```python
from build123d import *

# Parameters (mm, degrees)
SKETCH1_R           = 6
SKETCH1_R_2         = 1.1
BOSS_EXTRUDE1_DEPTH = 2.9
SKETCH2_R           = 6
CUT_EXTRUDE1_DEPTH  = 11.278132126
CUT_EXTRUDE2_DEPTH  = 2.8


with BuildPart() as part:
    # Sketch1 → Boss-Extrude1 (new, symmetric)
    with BuildSketch(Plane.XY):
        Circle(SKETCH1_R)
        Circle(SKETCH1_R_2, mode=Mode.SUBTRACT)
    extrude(amount=BOSS_EXTRUDE1_DEPTH, both=True)

    # Sketch2 → Cut-Extrude1 (cut, through all)
    with BuildSketch(Plane.XY.offset(2.9)):
        Circle(SKETCH2_R)
        with BuildLine():
            ThreePointArc((-0.904303163, 2.859411966), (-1.23929318, 3.784776039), (-2.052505646, 4.339034521))
            ThreePointArc((-2.052505646, 4.339034521), (-2.138842368, 4.297133152), (-2.224324134, 4.253514094))
            ThreePointArc((-2.224324134, 4.253514094), (-2.272407373, 3.270556831), (-1.736096974, 2.44539737))
            ThreePointArc((-1.736096974, 2.44539737), (-2.100579038, 2.140459929), (-2.412316811, 1.781776811))
            ThreePointArc((-2.412316811, 1.781776811), (-3.227244783, 2.333509881), (-4.210932449, 2.303920118))
            ThreePointArc((-4.210932449, 2.303920118), (-4.256151318, 2.219273746), (-4.29966888, 2.133740266))
            ThreePointArc((-4.29966888, 2.133740266), (-3.760801254, 1.310248516), (-2.841900466, 0.957915832))
            ThreePointArc((-2.841900466, 0.957915832), (-2.957534919, 0.496979078), (-2.998907428, 0.023563475))
            ThreePointArc((-2.998907428, 0.023563475), (-3.982498568, -0.009077739), (-4.760926181, -0.611213463))
            ThreePointArc((-4.760926181, -0.611213463), (-4.747755125, -0.706272801), (-4.732686255, -0.801049821))
            ThreePointArc((-4.732686255, -0.801049821), (-3.812696882, -1.150530198), (-2.862194572, -0.895456995))
            ThreePointArc((-2.862194572, -0.895456995), (-2.684812984, -1.336330888), (-2.440017337, -1.743650307))
            ThreePointArc((-2.440017337, -1.743650307), (-3.216573261, -2.348197971), (-3.49240793, -3.292884275))
            ThreePointArc((-3.49240793, -3.292884275), (-3.425877845, -3.362047143), (-3.357978338, -3.429866103))
            ThreePointArc((-3.357978338, -3.429866103), (-2.408271889, -3.171845481), (-1.789227635, -2.406795685))
            ThreePointArc((-1.789227635, -2.406795685), (-1.386583742, -2.659207876), (-0.949123556, -2.844848937))
            ThreePointArc((-0.949123556, -2.844848937), (-1.222026295, -3.79038639), (-0.889908552, -4.716785215))
            ThreePointArc((-0.889908552, -4.716785215), (-0.795431669, -4.733633748), (-0.700636829, -4.74859011))
            ThreePointArc((-0.700636829, -4.74859011), (-0.083968889, -3.981623598), (-0.032836554, -2.998820228))
            ThreePointArc((-0.032836554, -2.998820228), (0.44127336, -2.966357838), (0.904303163, -2.859411966))
            ThreePointArc((0.904303163, -2.859411966), (1.23929318, -3.784776039), (2.052505646, -4.339034521))
            ThreePointArc((2.052505646, -4.339034521), (2.138842368, -4.297133152), (2.224324134, -4.253514094))
            ThreePointArc((2.224324134, -4.253514094), (2.272407373, -3.270556831), (1.736096974, -2.44539737))
            ThreePointArc((1.736096974, -2.44539737), (2.100579038, -2.140459929), (2.412316811, -1.781776811))
            ThreePointArc((2.412316811, -1.781776811), (3.227244783, -2.333509881), (4.210932449, -2.303920118))
            ThreePointArc((4.210932449, -2.303920118), (4.256151318, -2.219273746), (4.29966888, -2.133740266))
            ThreePointArc((4.29966888, -2.133740266), (3.760801254, -1.310248516), (2.841900466, -0.957915832))
            ThreePointArc((2.841900466, -0.957915832), (2.957534919, -0.496979078), (2.998907428, -0.023563475))
            ThreePointArc((2.998907428, -0.023563475), (3.982498568, 0.009077739), (4.760926181, 0.611213463))
            ThreePointArc((4.760926181, 0.611213463), (4.747755125, 0.706272801), (4.732686255, 0.801049821))
            ThreePointArc((4.732686255, 0.801049821), (3.812696882, 1.150530198), (2.862194572, 0.895456995))
            ThreePointArc((2.862194572, 0.895456995), (2.684812984, 1.336330888), (2.440017337, 1.743650307))
            ThreePointArc((2.440017337, 1.743650307), (3.216573261, 2.348197971), (3.49240793, 3.292884275))
            ThreePointArc((3.49240793, 3.292884275), (3.425877845, 3.362047143), (3.357978338, 3.429866103))
            ThreePointArc((3.357978338, 3.429866103), (2.408271889, 3.171845481), (1.789227635, 2.406795685))
            ThreePointArc((1.789227635, 2.406795685), (1.386583742, 2.659207876), (0.949123556, 2.844848937))
            ThreePointArc((0.949123556, 2.844848937), (1.222026295, 3.79038639), (0.889908552, 4.716785215))
            ThreePointArc((0.889908552, 4.716785215), (0.795431669, 4.733633748), (0.700636829, 4.74859011))
            ThreePointArc((0.700636829, 4.74859011), (0.083968889, 3.981623598), (0.032836554, 2.998820228))
            ThreePointArc((0.032836554, 2.998820228), (-0.44127336, 2.966357838), (-0.904303163, 2.859411966))
        make_face(mode=Mode.SUBTRACT)
    extrude(amount=-CUT_EXTRUDE1_DEPTH, mode=Mode.SUBTRACT)

    # Sketch3 → Cut-Extrude2 (cut)
    with BuildSketch(Plane.XY.offset(2.9)):
        with BuildLine():
            ThreePointArc((0.700636829, 4.74859011), (0.083968889, 3.981623598), (0.032836554, 2.998820228))
            ThreePointArc((0.032836554, 2.998820228), (-0.44127336, 2.966357838), (-0.904303163, 2.859411966))
            ThreePointArc((-0.904303163, 2.859411966), (-1.23929318, 3.784776039), (-2.052505646, 4.339034521))
            ThreePointArc((-2.052505646, 4.339034521), (-2.138842368, 4.297133152), (-2.224324134, 4.253514094))
            ThreePointArc((-2.224324134, 4.253514094), (-2.272407373, 3.270556831), (-1.736096974, 2.44539737))
            ThreePointArc((-1.736096974, 2.44539737), (-2.100579038, 2.140459929), (-2.412316811, 1.781776811))
            ThreePointArc((-2.412316811, 1.781776811), (-3.227244783, 2.333509881), (-4.210932449, 2.303920118))
            ThreePointArc((-4.210932449, 2.303920118), (-4.256151318, 2.219273746), (-4.29966888, 2.133740266))
            ThreePointArc((-4.29966888, 2.133740266), (-3.760801254, 1.310248516), (-2.841900466, 0.957915832))
            ThreePointArc((-2.841900466, 0.957915832), (-2.957534919, 0.496979078), (-2.998907428, 0.023563475))
            ThreePointArc((-2.998907428, 0.023563475), (-3.982498568, -0.009077739), (-4.760926181, -0.611213463))
            ThreePointArc((-4.760926181, -0.611213463), (-4.747755125, -0.706272801), (-4.732686255, -0.801049821))
            ThreePointArc((-4.732686255, -0.801049821), (-3.812696882, -1.150530198), (-2.862194572, -0.895456995))
            ThreePointArc((-2.862194572, -0.895456995), (-2.684812984, -1.336330888), (-2.440017337, -1.743650307))
            ThreePointArc((-2.440017337, -1.743650307), (-3.216573261, -2.348197971), (-3.49240793, -3.292884275))
            ThreePointArc((-3.49240793, -3.292884275), (-3.425877845, -3.362047143), (-3.357978338, -3.429866103))
            ThreePointArc((-3.357978338, -3.429866103), (-2.408271889, -3.171845481), (-1.789227635, -2.406795685))
            ThreePointArc((-1.789227635, -2.406795685), (-1.386583742, -2.659207876), (-0.949123556, -2.844848937))
            ThreePointArc((-0.949123556, -2.844848937), (-1.222026295, -3.79038639), (-0.889908552, -4.716785215))
            ThreePointArc((-0.889908552, -4.716785215), (-0.795431669, -4.733633748), (-0.700636829, -4.74859011))
            ThreePointArc((-0.700636829, -4.74859011), (-0.083968889, -3.981623598), (-0.032836554, -2.998820228))
            ThreePointArc((-0.032836554, -2.998820228), (0.44127336, -2.966357838), (0.904303163, -2.859411966))
            ThreePointArc((0.904303163, -2.859411966), (1.23929318, -3.784776039), (2.052505646, -4.339034521))
            ThreePointArc((2.052505646, -4.339034521), (2.138842368, -4.297133152), (2.224324134, -4.253514094))
            ThreePointArc((2.224324134, -4.253514094), (2.272407373, -3.270556831), (1.736096974, -2.44539737))
            ThreePointArc((1.736096974, -2.44539737), (2.100579038, -2.140459929), (2.412316811, -1.781776811))
            ThreePointArc((2.412316811, -1.781776811), (3.227244783, -2.333509881), (4.210932449, -2.303920118))
            ThreePointArc((4.210932449, -2.303920118), (4.256151318, -2.219273746), (4.29966888, -2.133740266))
            ThreePointArc((4.29966888, -2.133740266), (3.760801254, -1.310248516), (2.841900466, -0.957915832))
            ThreePointArc((2.841900466, -0.957915832), (2.957534919, -0.496979078), (2.998907428, -0.023563475))
            ThreePointArc((2.998907428, -0.023563475), (3.982498568, 0.009077739), (4.760926181, 0.611213463))
            ThreePointArc((4.760926181, 0.611213463), (4.747755125, 0.706272801), (4.732686255, 0.801049821))
            ThreePointArc((4.732686255, 0.801049821), (3.812696882, 1.150530198), (2.862194572, 0.895456995))
            ThreePointArc((2.862194572, 0.895456995), (2.684812984, 1.336330888), (2.440017337, 1.743650307))
            ThreePointArc((2.440017337, 1.743650307), (3.216573261, 2.348197971), (3.49240793, 3.292884275))
            ThreePointArc((3.49240793, 3.292884275), (3.425877845, 3.362047143), (3.357978338, 3.429866103))
            ThreePointArc((3.357978338, 3.429866103), (2.408271889, 3.171845481), (1.789227635, 2.406795685))
            ThreePointArc((1.789227635, 2.406795685), (1.386583742, 2.659207876), (0.949123556, 2.844848937))
            ThreePointArc((0.949123556, 2.844848937), (1.222026295, 3.79038639), (0.889908552, 4.716785215))
            ThreePointArc((0.889908552, 4.716785215), (0.795431669, 4.733633748), (0.700636829, 4.74859011))
        make_face()
    extrude(amount=-CUT_EXTRUDE2_DEPTH, mode=Mode.SUBTRACT)


solid = part.part
```
Can you work these out from the model? Positions are in its coordinate system, mm. Coordinates: 2 decimals unless noted, no trailing zeros. Order: outer loops, then holes, each group sorted by start corner. A loop starts at its lowest first (then second) coordinate and runs counter-clockwise, first axis right, second up.
1. If we section it at B-B (x = 0.5): Please give me the cut outline in (y, z).
2. If we section it at C-C (y = -1.5): Please give me the cut outline in (x, z).
3. Thinking about a two-plate mould opening in Y: for faces 1 (the face through (-1, -1, -2.9)), 2 (the face through (1.392, 2.656, -1.379)), which applies, +Y half, -Y half, draft (parallel to the pull), parting line (faces both ways), or undercut?
4. If we section it at A-A (y = -0.5): Please give me the cut outline in (x, z).
5. I'm going to push a flat-ended pin straight in: pin 1 (3 mm diameter, centred on x = -1, y = 3.5, fed in from -Z). Where does the tip first touch, or does it pass through?
6. I need wall thicknesses on line 1 (X direction, y = 4, z = -0.9); line 2 (Y direction, x = 3.25, z = -1.15); line 3 (X direction, y = 2.5, z = -0.8). Which ranges of each line are inside material? Lowest first, please.
Entries:
1. outline: (-2.96, -2.9) - (-0.98, -2.9) - (-0.98, 0.1) - (-2.96, 0.1) - close; (0.98, -2.9) - (4.59, -2.9) - (4.59, 0.1) - (0.98, 0.1) - close
2. outline: (-2.6, -2.9) - (3.96, -2.9) - (3.96, 0.1) - (-2.6, 0.1) - close
3. face 1: draft
3. face 2: undercut
4. outline: (-4.68, -2.9) - (-0.98, -2.9) - (-0.98, 0.1) - (-4.68, 0.1) - close; (0.98, -2.9) - (2.96, -2.9) - (2.96, 0.1) - (0.98, 0.1) - close
5. pin 1: stops at z = -2.9
6. line 1: x = -2.3 to -1.44, 0.09 to 1.2
6. line 2: y = -2.34 to -1.03, -0.07 to 1.08, 2.4 to 3.43
6. line 3: x = -1.8 to 1.66, 1.83 to 3.31
